CAD build for the part. Positions are in the model's coordinates, mm. A direction names the side the tool comes from. Round coordinates to 2 decimals unless told otherwise and drop trailing zeros. Write each loop counter-clockwise with the first axis right and the second up, starting at its lowest first coordinate (ties: lowest second). Pieces come first, ordered by that corner, then holes. Notation, with made-up numbers: (88.25, 2.25) - (134.25, 2.25) arc R22 cw to (134.25, 30.25) - close; hole circle Ø2 at (37, 32). An arc over 180 degrees is marked (long way). Answer in a Markdown table with one row per item.
```python
from build123d import *

# Parameters (mm, degrees)
ESQUISSE1_R        = 2
ESQUISSE1_W        = 5
ESQUISSE1_H        = 5
BOSS_EXTRU_1_DEPTH = 5
CONG_1_R           = 5


with BuildPart() as part:
    # Esquisse1 → Boss.-Extru.1 (new body)
    with BuildSketch(Plane.XY):
        Polygon((15, 30), (15, 40), (105, 40), (105, 30), (120, 30), (120, 0), (105, 0), (105, -10), (15, -10), (-5.5, -10), (-5.5, 30), (0, 30), align=None)
        with Locations(Location((110, 15, 0), (0, 0, 180))):
            Circle(ESQUISSE1_R, mode=Mode.SUBTRACT)
        with Locations((4.5, 15)):
            Circle(ESQUISSE1_R, mode=Mode.SUBTRACT)
        with Locations((9.5, -1.5)):
            Circle(ESQUISSE1_R, mode=Mode.SUBTRACT)
        with Locations((85.5, 31.5)):
            Rectangle(ESQUISSE1_W, ESQUISSE1_H, mode=Mode.SUBTRACT)
        with Locations((34.5, 31.5)):
            Rectangle(ESQUISSE1_W, ESQUISSE1_H, mode=Mode.SUBTRACT)
        with Locations((85.5, -1.5)):
            Rectangle(ESQUISSE1_W, ESQUISSE1_H, mode=Mode.SUBTRACT)
        with Locations((34.5, -1.5)):
            Rectangle(ESQUISSE1_W, ESQUISSE1_H, mode=Mode.SUBTRACT)
        with Locations((98, -1.5)):
            Rectangle(ESQUISSE1_W, ESQUISSE1_H, mode=Mode.SUBTRACT)
        with Locations((98, 31.5)):
            Rectangle(ESQUISSE1_W, ESQUISSE1_H, mode=Mode.SUBTRACT)
        with Locations((2, -1.5)):
            Rectangle(ESQUISSE1_W, ESQUISSE1_H, mode=Mode.SUBTRACT)
        with Locations((17, -1.5)):
            Rectangle(ESQUISSE1_W, ESQUISSE1_H, mode=Mode.SUBTRACT)
    extrude(amount=BOSS_EXTRU_1_DEPTH)

    # Congé1
    cong_1_edges = [part.edges().sort_by_distance(p)[0] for p in [
        (105, -10, 2.5),
        (105, 0, 2.5),
        (120, 0, 2.5),
        (120, 30, 2.5),
        (105, 30, 2.5),
        (105, 40, 2.5),
        (15, 40, 2.5),
        (15, 30, 2.5),
        (-5.5, -10, 2.5),
        (-5.5, 30, 2.5),
    ]]
    fillet(cong_1_edges, radius=CONG_1_R - 0.0001)  # a hair under: the kernel refuses the full size


solid = part.part
```
Q1. Saw through at A-A on y = 15. List the corners of the cut face in (x, z).
Computed:
| item | result |
|---|---|
| outline | (-5.5, 0) - (2.5, 0) - (2.5, 5) - (-5.5, 5) - close; (6.5, 0) - (108, 0) - (108, 5) - (6.5, 5) - close; (112, 0) - (120, 0) - (120, 5) - (112, 5) - close |
Q2. Saw through at C-C on z = 3.8. Count the separate pieces of the cut face and the enclosed holes in it, then the cut area to 3 significant figures.
Computed:
| item | result |
|---|---|
| separate pieces | 1 |
| enclosed holes | 11 |
| area | 5,510 mm2 |
Q3. Flat gauge pins, fed straight in: pin 1 (3 mm diameter, centred on x = 110, y = 15, fed in from -Z); pin 2 (2.5 mm diameter, centred on y = 32.5, z = 2, fed in from -X). Where does each tip first touch, or does it go through?
Computed:
| item | result |
|---|---|
| pin 1 | passes through |
| pin 2 | stops at x = 13.31 |
Q4. 3-axis set-ups, long thin cutter, end or side, ignore diameter. For faces 1 (the flat face through (112, 30, 2)), 2 (the flat face through (2, 1, 2)): which of +Z, -Z, +X, -X, +Y, -Y reach the whole face in a straight line?
Computed:
| item | result |
|---|---|
| face 1 | +Z, -Z, +X, +Y |
| face 2 | +Z, -Z |
Q5. Pull direction X, two halves, no side cores. Call faces 3 (the cylindrical face through (14, 32, 3)), 4 (the cylindrical face through (103, 39, 3)), 5 (the flat face through (58, 15, 5)), 6 (the cylindrical face through (7.502, -1.412, 2.465)): released by +X, released by -X, zero draft, split by the parting line, or undercut.
Computed:
| item | result |
|---|---|
| face 3 | released by -X |
| face 4 | released by +X |
| face 5 | zero draft |
| face 6 | undercut |
Q6. Drill centre lines: line 1 (Y direction, x = 110, z = 2.75); line 2 (Y direction, x = 9.5, z = 3.4); line 3 (X direction, y = -5, z = 0.6). Where is each one in solid material? Low to high.
Computed:
| item | result |
|---|---|
| line 1 | y = 0 to 13, 17 to 30 |
| line 2 | y = -10 to -3.5, 0.5 to 30 |
| line 3 | x = -5.5 to 105 |
Q7. Saw through at B-B on y = -1.5. List the corners of the cut face in (x, z), then the cut area to 3 significant figures.
Computed:
| item | result |
|---|---|
| outline | (-5.5, 0) - (-0.5, 0) - (-0.5, 5) - (-5.5, 5) - close; (4.5, 0) - (7.5, 0) - (7.5, 5) - (4.5, 5) - close; (11.5, 0) - (14.5, 0) - (14.5, 5) - (11.5, 5) - close; (19.5, 0) - (32, 0) - (32, 5) - (19.5, 5) - close; (37, 0) - (83, 0) - (83, 5) - (37, 5) - close; (88, 0) - (95.5, 0) - (95.5, 5) - (88, 5) - close; (100.5, 0) - (106.43, 0) - (106.43, 5) - (100.5, 5) - close |
| area | 415 mm2 |
